For this review, take the finished solid that the model builds, in its own axes (mm). Coordinates: 2 decimals unless noted, no trailing zeros. Loops run counter-clockwise (first coordinate to the right, second up) from the corner with the lowest first, then second, coordinate; pieces in that order, holes last. Notation, with made-up numbers: (74.5, -33) - (87.5, -33) arc R12 ccw to (87.5, -21) - close; hole circle Ø8 at (-0.5, -18.5). An arc over 180 degrees is marked (long way). Answer as a JSON object with one key per item and string values. Group by question number.
Item 1: We need section A-A (z = -94). Give the boundary of the cut face in (x, y).
Item 2: Clearance check with flat-ended pins moving along their axes: pin 1 (0.9 mm diameter, centred on x = -128.5, y = 1.5, fed in from -Z); pin 2 (1.5 mm diameter, centred on x = -175.5, y = 1.5, fed in from -Z); pin 3 (0.9 mm diameter, centred on x = -13, y = 1.5, fed in from -Z). State where each tip first meets the part, or that it passes through.
Item 3: We need section B-B (x = -67.5). Give the boundary of the cut face in (y, z).
Item 4: We need section D-D (y = 1.1). State how many separate pieces and enclosed holes the cut face has, then the cut area to 3 significant figures.
Item 5: We need section C-C (z = -178.5). Give the boundary of the cut face in (x, y), then the cut area to 3 significant figures.
Item 6: To check wall thickness, follow line 1 (X direction, y = 0.85, z = -98); line 2 (Z direction, x = -11.5, y = 2.2); line 3 (X direction, y = 1.35, z = -83.5). State the ranges of each line that lie inside material, in increasing order.
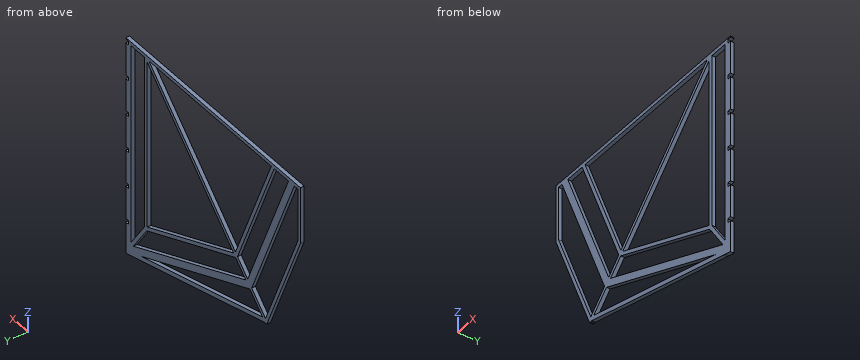
Autodesk Inventor part; units mm, degrees
ref_plane "YZ Plane" through (0, 0, 0) normal (1, 0, 0) x (0, 1, 0)
ref_plane "XZ Plane" through (0, 0, 0) normal (0, 1, 0) x (-1, 0, 0)
ref_plane "XY Plane" through (0, 0, 0) normal (0, 0, 1) x (1, 0, 0)
sketch "草圖1" plane through (0, 0, 0) normal (0, 1, 0) x (-1, 0, 0)
  line L0 (0, 0) -> (0, -200)
  line L1 (0, 0) -> (200, 0)
  line L2 (0, 0) -> (141.4214, -141.4214)
  line L3 (200, 0) -> (141.4214, -141.4214)
  line L4 (141.4214, -141.4214) -> (0, -200)
  line L5 (191.0204, -6) -> (6, -6)
  line L6 (6, -6) -> (6, -191.0204)
  line L7 (6, -191.0204) -> (136.8292, -136.8292)
  line L8 (136.8292, -136.8292) -> (191.0204, -6)
  line L9 (2.1213, 0) -> (142.0427, -139.9214)
  line L10 (0, -2.1213) -> (139.9214, -142.0427)
  line L11 (168.5713, -21) -> (21, -21)
  line L12 (21, -21) -> (21, -168.5713)
  line L13 (21, -168.5713) -> (125.3487, -125.3487)
  line L14 (125.3487, -125.3487) -> (168.5713, -21)
  line L15 (164.0815, -24) -> (24, -24)
  line L16 (24, -24) -> (24, -164.0815)
  line L17 (24, -164.0815) -> (123.0526, -123.0526)
  line L18 (123.0526, -123.0526) -> (164.0815, -24)
  line L19 (191.0204, -6) -> (168.5713, -21)
  line L20 (191.8537, -7.2472) -> (169.4046, -22.2472)
  line L21 (190.187, -4.7528) -> (167.7379, -19.7528)
  line L22 (167.7379, -19.7528) -> (161.3815, -24)
  line L23 (169.4046, -22.2472) -> (163.0482, -26.4944)
  line L24 (24, -164.0815) -> (6, -191.0204)
  line L25 (25.2472, -164.9148) -> (7.2472, -191.8537)
  line L26 (22.7528, -163.2481) -> (4.7528, -190.187)
  line L27 (175, 0) -> (171.8, 0)
  line L28 (171.8, 0) -> (171.8, -3)
  line L29 (171.8, -3) -> (175, -3)
  line L30 (175, -3) -> (175, 0)
  line L31 (141.8, -3) -> (145, -3)
  line L32 (141.8, 0) -> (141.8, -3)
  line L33 (145, -3) -> (145, 0)
  line L34 (111.8, -3) -> (115, -3)
  line L35 (111.8, 0) -> (111.8, -3)
  line L36 (115, -3) -> (115, 0)
  line L37 (81.8, -3) -> (85, -3)
  line L38 (81.8, 0) -> (81.8, -3)
  line L39 (85, -3) -> (85, 0)
  line L40 (51.8, -3) -> (55, -3)
  line L41 (51.8, 0) -> (51.8, -3)
  line L42 (55, -3) -> (55, 0)
  line L43 (21.8, -3) -> (25, -3)
  line L44 (21.8, 0) -> (21.8, -3)
  line L45 (25, -3) -> (25, 0)
  line L46 (0, -200) -> (0, -222)
  line L47 (0, -222) -> (156.9777, -156.9777)
  line L48 (200, 0) -> (222, 0)
  line L49 (141.4214, -141.4214) -> (156.9777, -156.9777)
  line L50 (222, 0) -> (156.9777, -156.9777)
  line L51 (197.0204, 0) -> (197.0204, -60.3062)
  line L52 (0, -222) -> (0, -225)
  line L53 (0, -225) -> (159.099, -159.099)
  line L54 (156.9777, -156.9777) -> (159.099, -159.099)
  line L55 (159.099, -159.099) -> (225, 0)
  line L56 (222, 0) -> (225, 0)
  line L57 (197.0204, -60.3062) -> (197.0204, -67.5488)
  line L58 (0, -200) -> (0, -222)
  line L59 (6, -197.5147) -> (6, -219.5147)
  line L60 (194.0204, -67.5488) -> (194.0204, -14.4361)
  line L61 (142.0427, -139.9214) -> (157.599, -155.4777)
  line L62 (139.9214, -142.0427) -> (157.599, -159.7203)
  line L63 (0, -22) -> (3, -22)
  line L64 (3, -22) -> (3, -25.2)
  line L65 (3, -25.2) -> (0, -25.2)
  line L66 (0, -25.2) -> (0, -22)
  line L67 (3, -52) -> (3, -55.2)
  line L68 (0, -52) -> (3, -52)
  line L69 (3, -55.2) -> (0, -55.2)
  line L70 (3, -82) -> (3, -85.2)
  line L71 (0, -82) -> (3, -82)
  line L72 (3, -85.2) -> (0, -85.2)
  line L73 (3, -112) -> (3, -115.2)
  line L74 (0, -112) -> (3, -112)
  line L75 (3, -115.2) -> (0, -115.2)
  line L76 (3, -142) -> (3, -145.2)
  line L77 (0, -142) -> (3, -142)
  line L78 (3, -145.2) -> (0, -145.2)
  line L79 (3, -172) -> (3, -175.2)
  line L80 (0, -172) -> (3, -172)
  line L81 (3, -175.2) -> (0, -175.2)
  line L82 (21, -21) -> (24, -21)
  line L83 (24, -21) -> (24, -6)
  line L84 (24, -6) -> (21, -6)
  line L85 (21, -6) -> (21, -21)
  line L86 (21, -168.5713) -> (21, -213.3015)
  line L87 (24, -164.0815) -> (24, -212.0589)
  line L88 (21, -213.3015) -> (21, -216.3015)
  line L89 (24, -212.0589) -> (24, -215.0589)
  line L90 (21, -6) -> (21, 0)
  line L91 (168.5713, -21) -> (213.3015, -21)
  line L92 (164.0815, -24) -> (212.0589, -24)
  line L93 (212.0589, -24) -> (215.0589, -24)
  line L94 (213.3015, -21) -> (216.3015, -21)
  line L95 (21, -21) -> (0, -21)
  line L96 (24, -24) -> (6, -24)
  line L97 (6, -197.5147) -> (155.4777, -157.599)
  line L98 (155.9937, -159.5313) -> (8, -199.0507)
  line L99 (8, -199.0507) -> (8, -219.5147)
  line L100 (155.0907, -156.1498) -> (4.5, -196.3627)
  line L101 (4.5, -196.3627) -> (4.5, -219.5147)
  line L102 (155.9937, -159.5313) -> (158.7857, -158.7857)
  line L103 (8, -199.0507) -> (6, -199.5848)
  line L104 (6, -199.5848) -> (0, -201.187)
  point P0 (8.1213, -6)
  point P1 (137.4505, -135.3292)
  point P2 (135.3292, -137.4505)
  point P3 (6, -8.1213)
  point P4 (121.5526, -123.6739)
  point P5 (24, -26.1213)
  point P6 (21, -23.1213)
  point P7 (123.8487, -125.97)
  point P8 (123.6739, -121.5526)
  point P9 (125.97, -123.8487)
  point P10 (23.1213, -21)
  point P11 (26.1213, -24)
  point P12 (21, -165.8714)
  point P13 (6, -188.3204)
  point P14 (8.4944, -189.9871)
  point P15 (23.4944, -167.5381)
  point P16 (188.3204, -6)
  point P17 (165.8714, -21)
  point P18 (167.5381, -23.4944)
  point P19 (189.9871, -8.4944)
  point P20 (171.8, 0)
  point P21 (141.8, 0)
  point P22 (111.8, 0)
  point P23 (81.8, 0)
  point P24 (51.8, 0)
  point P25 (21.8, 0)
  point P26 (156.9777, -156.9777)
  point P27 (197.0204, -7.1935)
  point P28 (157.5991, -156.7203)
  point P29 (0, -25.2)
  point P30 (0, -55.2)
  point P31 (0, -85.2)
  point P32 (0, -115.2)
  point P33 (0, -145.2)
  point P34 (0, -175.2)
  point P35 (167.3286, -24)
  point P36 (183.5645, -24)
  point P37 (190.0589, -24)
  point P38 (194.0204, -24)
  point P39 (197.0204, -21)
  point P40 (21, -24)
  point P41 (21, -21)
  point P42 (154.2524, -156.3737)
  point P43 (16.5488, -193.1453)
  point P44 (157.1115, -159.2328)
  point P45 (0, -201.187)
  dimension "d0" = 200
  dimension "d1" = 200
  dimension "d2" = 45
  dimension "d3" = 67.5
  dimension "d4" = 6
  dimension "d5" = 1.5
  dimension "d6" = 1.5
  dimension "d9" = 15
  dimension "d10" = 3
  dimension "d11" = 1.5
  dimension "d12" = 1.5
  dimension "d13" = 1.5
  dimension "d14" = 1.5
  dimension "d15" = 3
  dimension "d16" = 3.2
  dimension "d17" = 25
  dimension "d20" = 30
  dimension "d27" = 22
  dimension "d28" = 22
  dimension "d29" = 6
  dimension "d30" = 3
  dimension "d31" = 3
  dimension "d32" = 6
  dimension "d34" = 3
  dimension "d35" = 3
  dimension "d36" = 3.2
  dimension "d37" = 22
  dimension "d40" = 30
  dimension "d49" = 3
  dimension "d50" = 2
  dimension "d51" = 1.5
extrude "擠出1" add sketch "草圖1" along normal blind 3 contours L95 L6 L7 L86 L4 L100 L101 L0 L81 L79 L80 L78 L76 L77 L75 L73 L74 L72 L70 L71 L69 L67 L68 L65 L64 L63 | L11 L9 L15 L2 | L2 L96 L10 L12 | L12 L10 L95 | L95 L10 L12 L96 L6 | L15 L9 L18 L2 | L2 L17 L10 L16 | L16 L10 L96 | L11 L22 L15 L9 | L10 L96 L12 | L18 L9 L14 L2 | L2 L13 L10 L17 | L16 L24 L12 L96 L10 | L26 L12 L24 L6 | L14 L9 L8 L2 | L2 L7 L10 L13 | L10 L13 L87 L17 | L18 L23 L92 L14 L9 | L22 L11 L14 L23 L92 L15 | L87 L25 L13 L24 | L24 L86 L25 L7 | L8 L9 L3 L2 | L2 L4 L10 L7 | L18 L92 L23 | L13 L25 L86 | L87 L13 L25 | L91 L20 L23 L14 | L49 L47 L62 L4 | L3 L61 L50 L49 | L10 L4 L87 L7 | L8 L92 L3 L9 | L92 L23 L14 | L14 L23 L20 L91 L8 L92 | L7 L87 L4 L86 | L91 L3 L92 L8 | L54 L102 L62 L47 | L50 L57 L55 L54 | L91 L60 L92 L3 | L62 L97 L87 L100 | L62 L102 L98 L47 | L47 L98 L87 L97 | L54 L53 L62 L102 | L100 L86 L97 L4 | L4 L101 L100 | L100 L87 L97 L86 | L91 L51 L92 L60 | L92 L51 L50 L60 | L87 L98 L86 L97 | L59 L104 L101 L4 | L97 L86 L98 L103 L59 | L101 L104 L46 L4
sketch "草圖2" plane through (-3, 0, -25.2) normal (0, 0, 1) x (1, 0, 0)
  line L0 (0, 0) -> (0, 3)
  line L1 (-154.599, 3) -> (-156.099, 3)
  line L2 (0, 0) -> (-3, 0)
  line L3 (-3, 0) -> (-3, 3)
  line L4 (-3, 3) -> (0, 3)
  line L5 (0, 3) -> (0, 0)
  circle A0 centre (-1.5, 1.5) radius 2.1213
  point P0 (3, 0)
  point P1 (3, 3)
  dimension "d45" = 3
  dimension "d46" = 4.2426
properties part number "side_sail_2"
Check sheet entries:
{
 "1": {"outline": "(-186.06, 0) - (-183.06, 0) - (-183.06, 3) - (-186.06, 3) - close; (-161.06, 0) - (-154.57, 0) - (-154.57, 3) - (-161.06, 3) - close; (-138.33, 0) - (-135.09, 0) - (-135.09, 3) - (-138.33, 3) - close; (-96.12, 0) - (-91.88, 0) - (-91.88, 3) - (-96.12, 3) - close; (-24, 0) - (-21, 0) - (-21, 3) - (-24, 3) - close; (-6, 0) - (0, 0) - (0, 3) - (-6, 3) - close"},
 "2": {"pin 1": "stops at z = -166.99", "pin 2": "stops at z = -121.31", "pin 3": "stops at z = -197.84"},
 "3": {"outline": "(0, -183.16) - (3, -183.16) - (3, -179.54) - (0, -179.54) - close; (0, -172.04) - (3, -172.04) - (3, -165.55) - (0, -165.55) - close; (0, -149.31) - (3, -149.31) - (3, -146.06) - (0, -146.06) - close; (0, -69.62) - (3, -69.62) - (3, -65.38) - (0, -65.38) - close; (0, -24) - (3, -24) - (3, -21) - (0, -21) - close"},
 "4": {"separate pieces": "1", "enclosed holes": "7", "area": "5,840 mm2"},
 "5": {"outline": "(-84.96, 0) - (-71.39, 0) - (-71.39, 3) - (-84.96, 3) - close; (-51.91, 0) - (-36.23, 0) - (-36.23, 3) - (-51.91, 3) - close; (-16.17, 0) - (-12.56, 0) - (-12.56, 3) - (-16.17, 3) - close; (-6, 0) - (0, 0) - (0, 3) - (-6, 3) - close", "area": "117 mm2"},
 "6": {"line 1": "x = -184.41 to -181.41, -159.41 to -152.91, -136.68 to -133.43, -100.12 to -95.88, -24 to -21, -6 to 0", "line 2": "z = -198.12 to -188.74, -185.49 to -180.09, -24 to -21", "line 3": "x = -190.41 to -187.41, -165.41 to -158.92, -142.68 to -139.44, -85.62 to -81.38, -24 to -21, -6 to -3"}
}
